Answer from the drawing. Dimensions are ordinates in mm from the lowest x, y and z of the part. Coordinates: 2 decimals unless noted, no trailing zeros. Order: outer loops, then holes, each group sorted by start corner. A loop starts at its lowest first (then second) coordinate and runs counter-clockwise, first axis right, second up. Notation, with made-up numbers: (64, 29.25) -> (80, 29.25) arc R20 ccw to (80, 55.25) -> close; hole circle Ø1 at (-28.5, 36.25). An arc over 180 degrees is marked (long way). Answer in a Markdown table with one row per item.
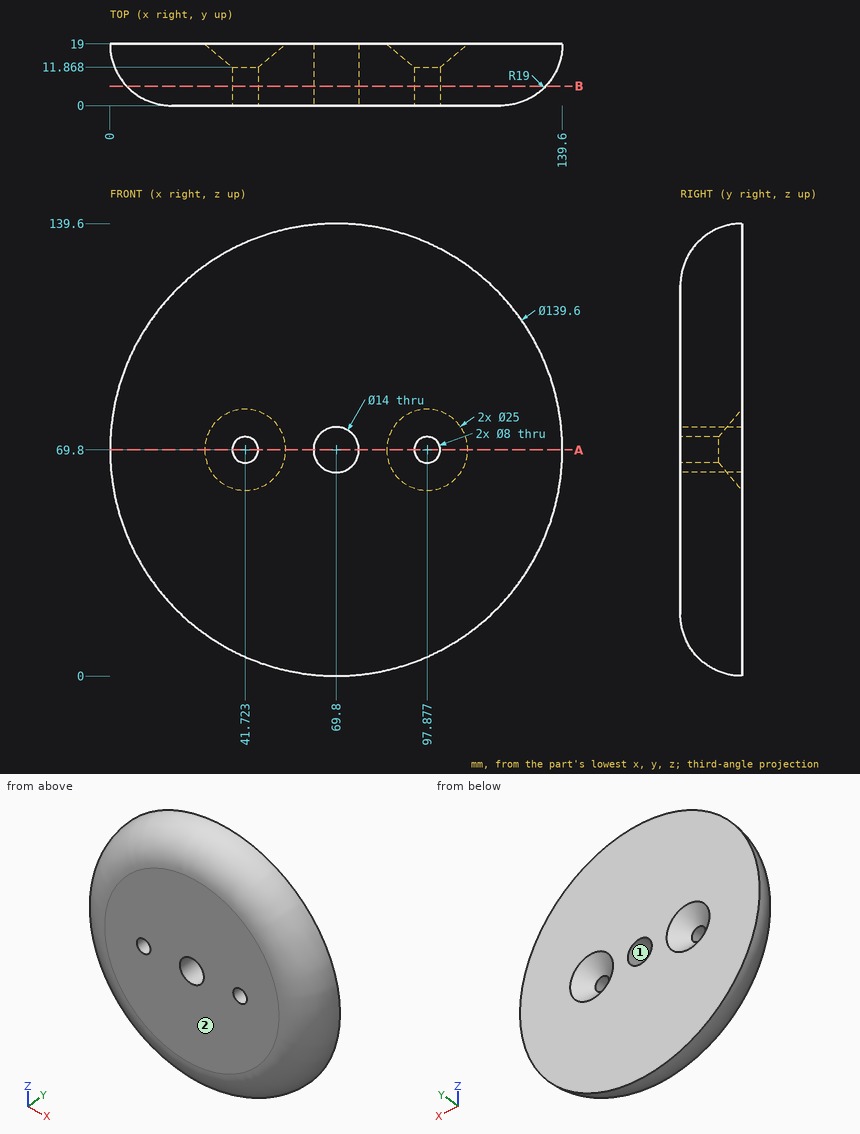
Q1. The part is cut by section B-B (y = 6). Write down the section's boundary in (x, z).
Outcome:
| item | result |
|---|---|
| outline | circle Ø129.31 at (69.8, 69.8); hole circle Ø8 at (41.72, 69.8); hole circle Ø14 at (69.8, 69.8); hole circle Ø8 at (97.88, 69.8) |
Q2. The part is cut by section A-A (z = 69.8). Give the number of separate pieces and of enclosed holes in the cut face, then the cut area to 3 significant figures.
Outcome:
| item | result |
|---|---|
| separate pieces | 4 |
| enclosed holes | 0 |
| area | 1,810 mm² |
Q3. Given pin 1 (1.5 mm diameter, centred on y = 7.5, z = 62.5, fed in from -X); pin 2 (13 mm diameter, centred on x = 41.72, z = 69.8, fed in from +Y); pin 3 (1.5 mm diameter, centred on y = 10.5, z = 60, fed in from -X), each flat-ended and moving along its own axis, determine where each tip first touches the part or whether it passes through.
Outcome:
| item | result |
|---|---|
| pin 1 | x = 3.73 |
| pin 2 | y = 13.97 |
| pin 3 | x = 2.34 |
Q4. For a pull along Z with two mould halves and no side action, classify the marked faces 1 and 2 as pulls with the +Z half, pulls with the -Z half, needs draft (parallel to the pull), parting line crosses it, or undercut.
Outcome:
| item | result |
|---|---|
| face 1 | undercut |
| face 2 | needs draft |
Q5. Consider line 1 (Z direction, x = 50, y = 10.25) (1 decimal); line 2 (X direction, y = 17.5, z = 94); line 3 (Y direction, x = 124.5, z = 99) (1 decimal). Determine where each line is inside the solid, lowest interval first.
Outcome:
| item | result |
|---|---|
| line 1 | 5.1 to 134.5 |
| line 2 | 4.39 to 135.21 |
| line 3 | 3.7 to 19 |
